For this review, use the dimensioned drawing (mm, ordinates from the lowest corner) and the shaded views. Coordinates: 2 decimals unless noted, no trailing zeros. Write each loop counter-clockwise with the first axis right and the second up, starting at its lowest first coordinate (ties: lowest second). Pieces come first, ordered by that corner, then holes.
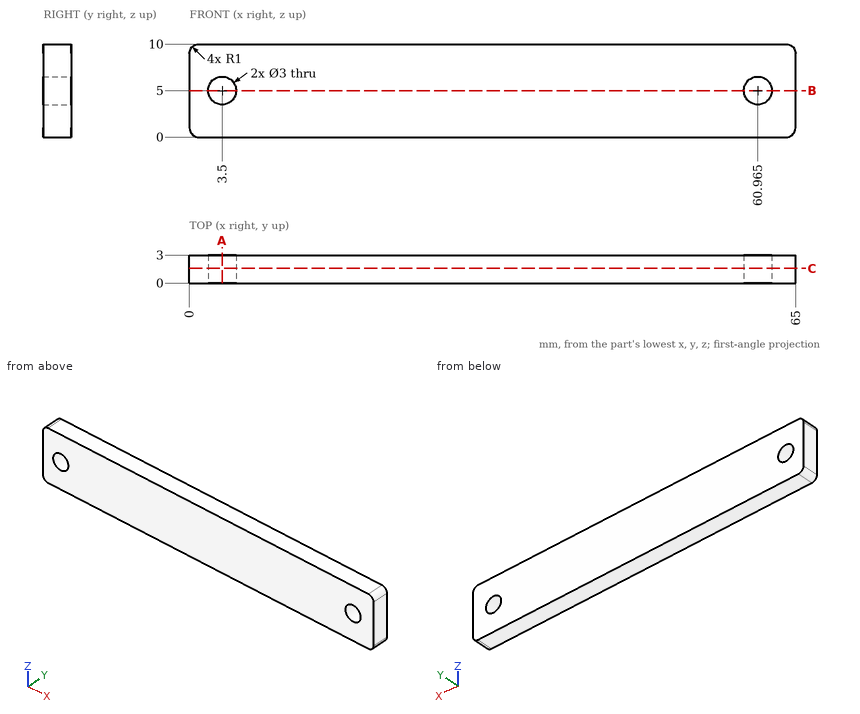
Item 1: Take a section at B-B, the plane z = 5. Write out the cut boundary in (x, y) (1 decimal), plus the area to 3 significant figures.
Solved:
outline: (0, 0) - (2, 0) - (2, 3) - (0, 3) - close; (5, 0) - (59.5, 0) - (59.5, 3) - (5, 3) - close; (62.5, 0) - (65, 0) - (65, 3) - (62.5, 3) - close
area: 177 mm2
Item 2: To check wall thickness, follow line 1 along X through (y, z) = (1.8, 5) (1 decimal); line 2 along Z through (x, y) = (3.5, 1.1); line 3 along Z through (x, y) = (60, 1.4). State the ranges of each line that lie inside material, in increasing order.
Solved:
line 1: x = 0 to 2, 5 to 59.5, 62.5 to 65
line 2: z = 0 to 3.5, 6.5 to 10
line 3: z = 0 to 3.85, 6.15 to 10
Item 3: For pin 1 (4 mm diameter, centred on x = 60.96, z = 5, fed in from -Y); pin 2 (1.8 mm diameter, centred on x = 3.5, z = 5, fed in from +Y), all flat-tipped, find the tip position at first contact; note any pin that passes through.
Solved:
pin 1: stops at y = 0
pin 2: passes through
Item 4: Take a section at A-A, the plane x = 3.5. Write out the cut boundary in (y, z), plus the area to 3 significant figures.
Solved:
outline: (0, 0) - (3, 0) - (3, 3.5) - (0, 3.5) - close; (0, 6.5) - (3, 6.5) - (3, 10) - (0, 10) - close
area: 21.0 mm2
Item 5: Take a section at C-C, the plane y = 1.6. Write out the cut boundary in (x, z) (1 decimal), plus the area to 3 significant figures.
Solved:
outline: (0, 1) arc R1 ccw to (1, 0) - (64, 0) arc R1 ccw to (65, 1) - (65, 9) arc R1 ccw to (64, 10) - (1, 10) arc R1 ccw to (0, 9) - close; hole circle Ø3 at (3.5, 5); hole circle Ø3 at (61, 5)
area: 635 mm2
